Read the model definition and answer for the solid it produces. Units are mm, in the model's axes. Face numbers are marked on the shaded views. A direction names the side the tool comes from. Coordinates: 2 decimals unless noted, no trailing zeros. Write each loop counter-clockwise with the first axis right and the second up, starting at its lowest first coordinate (ties: lowest second). Pieces come first, ordered by that corner, then holes.
from build123d import *

# Parameters (mm, degrees)
CROQUIS1_W              = 84.92
CROQUIS1_H              = 56
SALIENTE_EXTRUIR1_DEPTH = 1.33
REDONDEO1_R             = 6
CROQUIS2_R              = 1.375
CORTAR_EXTRUIR1_DEPTH   = 1.33
SALIENTE_EXTRUIR2_DEPTH = 13.5


with BuildPart() as part:
    # Croquis1 → Saliente-Extruir1 (new body)
    with BuildSketch(Plane(origin=(0, 0, 0), x_dir=(1, 0, 0), z_dir=(0, 1, 0))):
        Rectangle(CROQUIS1_W, CROQUIS1_H)
    extrude(amount=SALIENTE_EXTRUIR1_DEPTH)

    # Redondeo1
    redondeo1_edges = [part.edges().sort_by_distance(p)[0] for p in [
        (42.46, 0.665, 28),
        (-42.46, 0.665, 28),
        (-42.46, 0.665, -28),
        (42.46, 0.665, -28),
    ]]
    fillet(redondeo1_edges, radius=REDONDEO1_R)

    # Croquis2 → Cortar-Extruir1 (cut)
    with BuildSketch(Plane(origin=(0, 1.33, 0), x_dir=(1, 0, 0), z_dir=(0, 1, 0))):
        with Locations((-38.46, 24.5)):
            Circle(CROQUIS2_R)
        with Locations((-38.46, -24.5)):
            Circle(CROQUIS2_R)
        with Locations((19.54, -24.5)):
            Circle(CROQUIS2_R)
        with Locations((19.54, 24.5)):
            Circle(CROQUIS2_R)
    extrude(amount=-CORTAR_EXTRUIR1_DEPTH, mode=Mode.SUBTRACT)

    # Croquis3 → Saliente-Extruir2 (add)
    with BuildSketch(Plane(origin=(0, 1.33, 0), x_dir=(1, 0, 0), z_dir=(0, 1, 0))):
        Polygon((45.46, -18.762058392), (45.46, -19.412058392), (44.96, -19.412058392), (44.96, -18.762058392), (27.76, -18.762058392), (27.76, -5.362058392), (44.96, -5.362058392), (44.96, -4.712058392), (45.46, -4.712058392), (45.46, -5.362058392), align=None)
    extrude(amount=SALIENTE_EXTRUIR2_DEPTH)


solid = part.part
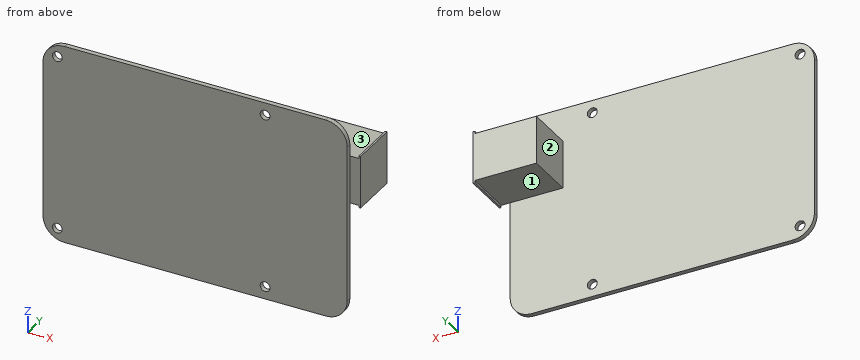
Item 1: The part is cut by section C-C (z = 16). Give the vertices of the cut face in (x, y), and give its area (3 significant figures).
Item 2: The part is cut by section D-D (y = 7). Give the vertices of the cut face in (x, z), and give its area (3 significant figures).
Item 3: For the marked faces 1, 2 and 3, determine the directions among +Z, -Z, +X, -X, +Y, -Y from which every point of the face is accessible in a straight line to the end or side of a thin tool.
Item 4: The part is cut by section B-B (z = 24.5). Give the vertices of the cut face in (x, y) (3 decimals).
Item 5: Find the intervals of material crossed by probe 1 along Z at (x, y) = (19.54, 0.55) (3 decimals); probe 2 along Z at (x, y) = (-38.46, 0.9) (3 decimals); probe 3 along X at (y, z) = (0.55, 24.5) (3 decimals), in increasing order.
Item 6: The part is cut by section A-A (x = 19.54). Give the vertices of the cut face in (y, z) (3 decimals), and give its area (3 significant figures).
Item 7: Given pin 1 (1.1 mm diameter, centred on y = 1, z = 3, fed in from +X); pin 2 (3 mm diameter, centred on x = 19.54, z = 24.5, fed in from +Y); pin 3 (7 mm diameter, centred on x = 37.5, y = 10.5, fed in from +Z), each flat-ended and moving along its own axis, determine where each tip first touches the part or whether it passes through.
Answer:
1. outline: (-42.46, 0) - (42.46, 0) - (42.46, 1.33) - (45.46, 1.33) - (45.46, 14.83) - (27.76, 14.83) - (27.76, 1.33) - (-42.46, 1.33) - close
1. area: 352 mm2
2. outline: (27.76, 5.36) - (44.96, 5.36) - (44.96, 4.71) - (45.46, 4.71) - (45.46, 19.41) - (44.96, 19.41) - (44.96, 18.76) - (27.76, 18.76) - close
2. area: 238 mm2
3. face 1: -Z, -X, +Y
3. face 2: +Z, -Z, -X, +Y
3. face 3: +Z, -X, +Y
4. outline: (-41.914, 0) - (-39.835, 0) - (-39.835, 1.33) - (-41.914, 1.33) - close; (-37.085, 0) - (18.165, 0) - (18.165, 1.33) - (-37.085, 1.33) - close; (20.915, 0) - (41.914, 0) - (41.914, 1.33) - (20.915, 1.33) - close
5. probe 1: z = -28 to -25.875, -23.125 to 23.125, 25.875 to 28
5. probe 2: z = -27.657 to -25.875, -23.125 to 23.125, 25.875 to 27.657
5. probe 3: x = -41.914 to -39.835, -37.085 to 18.165, 20.915 to 41.914
6. outline: (0, -28) - (1.33, -28) - (1.33, -25.875) - (0, -25.875) - close; (0, -23.125) - (1.33, -23.125) - (1.33, 23.125) - (0, 23.125) - close; (0, 25.875) - (1.33, 25.875) - (1.33, 28) - (0, 28) - close
6. area: 67.2 mm2
7. pin 1: stops at x = 42.46
7. pin 2: stops at y = 1.33
7. pin 3: stops at z = 18.76
